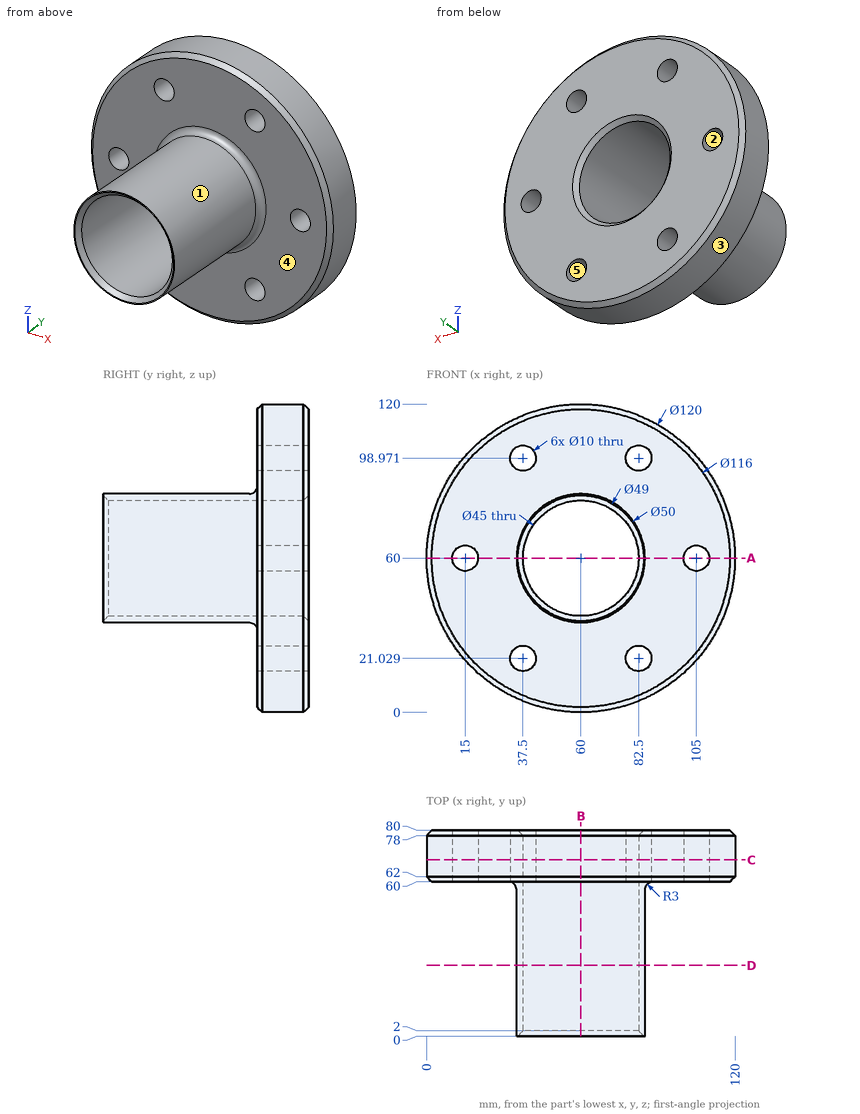
Check sheet for the drawn part. Datum: minimum x, y, z corner. Units: mm. A direction names the side the tool comes from. Round coordinates to 2 decimals unless told otherwise and drop trailing zeros. Order: outer loops, then holes, each group sorted by start corner. A loop starts at its lowest first (then second) coordinate and runs counter-clockwise, first axis right, second up.
1. Section check B-B on x = 60. Record the cut outline in (y, z), then the cut area to 3 significant figures.
Final values:
outline: (0, 35) - (57, 35) arc R3 cw to (60, 32) - (60, 2) - (62, 0) - (78, 0) - (80, 2) - (80, 35.5) - (78, 37.5) - (2, 37.5) - (0, 35.5) - close; (0, 84.5) - (2, 82.5) - (78, 82.5) - (80, 84.5) - (80, 118) - (78, 120) - (62, 120) - (60, 118) - (60, 88) arc R3 cw to (57, 85) - (0, 85) - close
area: 1,790 mm2
2. Access from +Z, -Z, +X, -X, +Y, -Y to the whole of each face (thin tool, end or side, straight path). Record for the marked faces 1 and 2.
Final values:
face 1: -Y
face 2: +Y, -Y
3. Release check for a two-part mould opening along X. For the marked faces 3, 4 and 5 record: +X half, -X half, draft (parallel to the pull), parting line (faces both ways), or undercut.
Final values:
face 3: parting line
face 4: draft
face 5: undercut
4. Section check D-D on y = 27.5. Record the cut outline in (x, z), then the cut area to 3 significant figures.
Final values:
outline: circle Ø50 at (60, 60); hole circle Ø45 at (60, 60)
area: 373 mm2
5. Section check C-C on y = 68.5. Record the cut outline in (x, z), then the cut area to 3 significant figures.
Final values:
outline: circle Ø120 at (60, 60); hole circle Ø10 at (15, 60); hole circle Ø10 at (37.5, 21.03); hole circle Ø10 at (37.5, 98.97); hole circle Ø45 at (60, 60); hole circle Ø10 at (82.5, 21.03); hole circle Ø10 at (82.5, 98.97); hole circle Ø10 at (105, 60)
area: 9,250 mm2
6. Section check A-A on z = 60. State how many separate pieces and enclosed holes the cut face has, then the cut area to 3 significant figures.
Final values:
separate pieces: 4
enclosed holes: 0
area: 1,390 mm2
7. Go/stop test with flat-tipped pins: P1, Ø8, axis at x = 37.5, z = 21.03, coming from the -Y side; P2, Ø1, axis at x = 50.5, z = 27, coming from the -Y side; P3, Ø6, axis at y = 34.5, z = 54, coming from the +X side; P4, Ø3, axis at x = 84.5, y = 14, coming from the -Z side. Record where each tip stops, or that it passes through.
Final values:
P1: passes through
P2: stops at y = 60
P3: stops at x = 84.82
P4: stops at z = 50.2
8. Thickness scan on L1, parallel to X at y = 73, z = 60; L2, parallel to X at y = 42, z = 60; L3, parallel to X at y = 70, z = 102.5. Record the ranges inside material, lowest first.
Final values:
L1: x = 0 to 10, 20 to 37.5, 82.5 to 100, 110 to 120
L2: x = 35 to 37.5, 82.5 to 85
L3: x = 17.65 to 33.96, 41.04 to 78.96, 86.04 to 102.35
